Can you work these out from the model? Positions are in its coordinate system, mm. Face numbers are marked on the shaded views. A direction names the side the tool comes from. Give positions to 0.01 mm unless a question says otherwise; leave off trailing zeros. Write each loop counter-clockwise with the first axis right and the second up, starting at its lowest first coordinate (ties: lowest second). Pieces come first, ordered by that corner, then holes. Notation, with made-up numbers: (68, 65) - (103, 65) arc R10 ccw to (103, 78) - close; hole circle Ø11 at (69.25, -20). An arc over 180 degrees is marked (long way). Use a Markdown table: item, result. Add a question column.
```python
from build123d import *

# Parameters (mm, degrees)
F0_W     = 320
F0_H     = 370
F1_DEPTH = 70
F2_W     = 254.012
F2_H     = 325.316
F3_DEPTH = 51
F4_W     = 342
F4_H     = 140
F5_DEPTH = 19


with BuildPart() as f1:
    # F0 (on Top) → F1 (new body)
    with BuildSketch(Plane.XY):
        Rectangle(F0_W, F0_H)
    extrude(amount=F1_DEPTH)

    # F2 (on face) → F3 (cut)
    with BuildSketch(Plane.XY.offset(70)):
        Rectangle(F2_W, F2_H)
    extrude(amount=-F3_DEPTH, mode=Mode.SUBTRACT)

    # F4 (on face) → F5 (join)
    with BuildSketch(Plane.XZ.offset(185)):
        with Locations((0, 29.569484)):
            Rectangle(F4_W, F4_H)
    extrude(amount=F5_DEPTH)


solid = f1.part
```
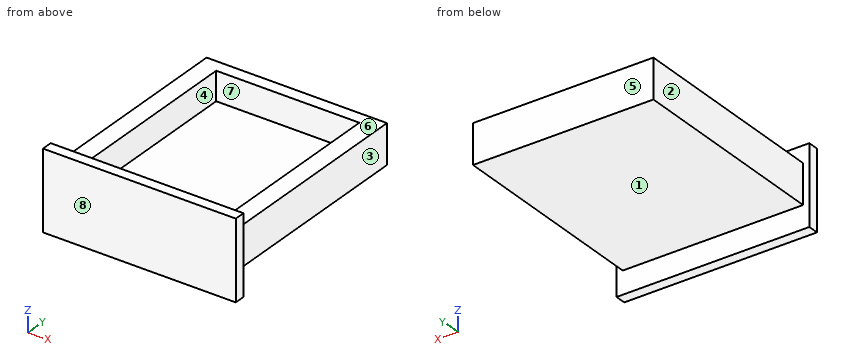
Q1. Suppose I cut it at B-B (z = 25.5). Please give me the cut outline in (x, y).
Q2. Suppose I cut it at C-C (y = -10). Please give me the cut outline in (x, z).
Q3. I'm going to push flat-ended pins straight in: P1, Ø10, axis at x = -34, y = -140, coming from the +Z side; P2, Ø21, axis at y = 24, z = 18, coming from the +X side; P3, Ø12, axis at y = 103, z = 55, coming from the -X side. Where does each tip first touch, or does it pass through?
Q4. If we mould it in two halves opening along Y, with no side actions, what happens to the marked faces 5, 6, 7 and 8? For each: released by +Y, released by -Y, zero draft, split by the parting line, or undercut.
Q5. On a 3-axis mill with a long thin cutter (end or side, diameter ignored), from which of +Z, -Z, +X, -X, +Y, -Y can I reach the whole of each face in a straight line? I mean the marked faces 1, 2, 3 and 4. Say none if no direction works.
Q6. Suppose I cut it at A-A (x = 143.5). Please give me the cut outline in (y, z), and give its area (3 significant figures).
Q7. Suppose I cut it at D-D (x = 85.5). Please give me the cut outline in (y, z).
Q8. If I drill on probe 1 along X at (y, z) = (-107, 26.5); probe 2 along Y at (x, z) = (-94.5, 57); probe 3 along Y at (x, z) = (-44, -8.5), over which ranges is the centre line in solid material (lowest first)? Write a range as [from, to].
Derived:
| question | item | result |
|---|---|---|
| 1 | outline | (-171, -204) - (171, -204) - (171, -185) - (160, -185) - (160, 185) - (-160, 185) - (-160, -185) - (-171, -185) - close; hole (-127.01, -162.66) - (127.01, -162.66) - (127.01, 162.66) - (-127.01, 162.66) - close |
| 2 | outline | (-160, 0) - (160, 0) - (160, 70) - (127.01, 70) - (127.01, 19) - (-127.01, 19) - (-127.01, 70) - (-160, 70) - close |
| 3 | P1 | z = 19 |
| 3 | P2 | x = 160 |
| 3 | P3 | x = -160 |
| 4 | face 5 | released by +Y |
| 4 | face 6 | zero draft |
| 4 | face 7 | undercut |
| 4 | face 8 | released by -Y |
| 5 | face 1 | -Z, +X, -X, +Y |
| 5 | face 2 | +Z, -Z, -X, +Y |
| 5 | face 3 | +Z, -Z, +X, +Y |
| 5 | face 4 | +Z |
| 6 | outline | (-204, -40.43) - (-185, -40.43) - (-185, 0) - (185, 0) - (185, 70) - (-185, 70) - (-185, 99.57) - (-204, 99.57) - close |
| 6 | area | 28,600 mm² |
| 7 | outline | (-204, -40.43) - (-185, -40.43) - (-185, 0) - (185, 0) - (185, 70) - (162.66, 70) - (162.66, 19) - (-162.66, 19) - (-162.66, 70) - (-185, 70) - (-185, 99.57) - (-204, 99.57) - close |
| 8 | probe 1 | [-160, -127.01], [127.01, 160] |
| 8 | probe 2 | [-204, -162.66], [162.66, 185] |
| 8 | probe 3 | [-204, -185] |
